Autodesk Inventor part; units mm, degrees
ref_plane "YZ Plane" through (0, 0, 0) normal (1, 0, 0) x (0, 1, 0)
ref_plane "XZ Plane" through (0, 0, 0) normal (0, 1, 0) x (-1, 0, 0)
ref_plane "XY Plane" through (0, 0, 0) normal (0, 0, 1) x (1, 0, 0)
sketch "Sketch1" plane through (0, 0, 0) normal (0, 1, 0) x (-1, 0, 0)
  line L0 (-27.94, -43.053) -> (27.94, -43.053)
  line L1 (27.94, -43.053) -> (27.94, 43.053)
  line L2 (27.94, 43.053) -> (-27.94, 43.053)
  line L3 (-27.94, 43.053) -> (-27.94, -43.053)
  line L4 (-27.94, -43.053) -> (27.94, 43.053) construction
  line L5 (27.94, -43.053) -> (-27.94, 43.053) construction
  point P0 (0, 0)
  dimension "d0" = 86.106
  dimension "d1" = 55.88
extrude "Extrusion1" add sketch "Sketch1" along normal blind 0.8
fillet "Fillet1" radius 3.9688 4 edges at (27.94, 0.4, 43.053) (27.94, 0.4, -43.053) (-27.94, 0.4, -43.053) (-27.94, 0.4, 43.053)
sketch "Sketch2" plane through (0, 0.8, 0) normal (0, 1, 0) x (1, 0, 0)
  line L0 (7.5, -73.053) -> (-7.5, -73.053)
  line L1 (-7.5, -73.053) -> (-7.5, -13.053)
  line L2 (-7.5, -13.053) -> (7.5, -13.053)
  line L3 (7.5, -13.053) -> (7.5, -73.053)
  line L4 (-23.9712, -43.053) -> (23.9713, -43.053)
  line L5 (7.5, -73.053) -> (-7.5, -13.053) construction
  line L6 (-7.5, -73.053) -> (7.5, -13.053) construction
  point P0 (0, 0)
  point P1 (0, -43.053)
  point P2 (-7.5, -43.053)
  point P3 (7.5, -43.053)
  dimension "d5" = 15
  dimension "d6" = 60
extrude "Extrusion2" cut sketch "Sketch2" against normal blind 25.4 contours L4 L1 L2 L3
fillet "Fillet2" radius 1.5875 4 edges at (-7.5, 0.4, 13.053) (7.5, 0.4, 13.053) (-7.5, 0.4, 43.053) (7.5, 0.4, 43.053)
properties part number "led_ring_cover"
Input: part model. Units: mm. Frame: model coordinates. A direction names the side the tool comes from. Give positions to 0.01 mm unless a question says otherwise; leave off trailing zeros. Write each loop counter-clockwise with the first axis right and the second up, starting at its lowest first coordinate (ties: lowest second). Pieces come first, ordered by that corner, then holes. Notation, with made-up numbers: (14, 52.5) -> (58, 52.5) arc R16 ccw to (58, 77.5) -> close; hole circle Ø1 at (64, 3.5). An arc over 180 degrees is marked (long way). Use one line per item in the form item = value. Start each with the question number.
1) Set-up query: faces 5 (the flat face through (0, 0, 1)), 6 (the cylindrical face through (-7.047, 0.394, 13.53)). Return all of +Z, -Z, +X, -X, +Y, -Y with unobstructed straight access to the full face (end or side cutting, diameter ignored); none if empty.
2) Draft query along X for faces 1 (the cylindrical face through (-7.953, 0.394, 42.576)), 2 (the cylindrical face through (-26.81, 0.41, 41.86)), 3 (the cylindrical face through (26.75, 0.41, 41.92)), 4 (the flat face through (0, 0.8, 1)). Return one class per face: pulls with the +X half, pulls with the -X half, needs draft (parallel to the pull), parting line crosses it, or undercut.
3) Ray query, probe 1 along X at (y, z) = (0.15, 35.5); probe 2 along Z at (x, y) = (-3, 0.4); probe 3 along Z at (x, y) = (-25.5, 0.5). Return the intervals inside material, ascending. Write a range as from..to.
4) Section query A-A on z = 37. Return the cut outline in (x, y), then the cut area to 3 significant figures.
5) Pin query (flat end, axial travel): pin 1 (3 mm diameter, centred on x = 7, z = 32, fed in from -Y). Return the tip coordinate at first contact, or that it passes through.
6) Section query B-B on y = 0.55. Return the cut outline in (x, z) (1 decimal).
7) Section query C-C on x = 4. Return the cut outline in (y, z), then the cut area to 3 significant figures.
Outcome:
q1.face_5 = +Z, -Z, +X, -X, -Y
q1.face_6 = +Z, +Y, -Y
q2.face_1 = undercut
q2.face_2 = pulls with the -X half
q2.face_3 = pulls with the +X half
q2.face_4 = needs draft
q3.probe_1 = -27.94..-7.5, 7.5..27.94
q3.probe_2 = -43.05..13.05
q3.probe_3 = -42.75..42.75
q4.outline = (-27.94, 0) -> (-7.5, 0) -> (-7.5, 0.8) -> (-27.94, 0.8) -> close; (7.5, 0) -> (27.94, 0) -> (27.94, 0.8) -> (7.5, 0.8) -> close
q4.area = 32.7 mm^2
q5.pin_1 = 0
q6.outline = (-27.9, -39.1) arc R4 ccw to (-24, -43.1) -> (24, -43.1) arc R4 ccw to (27.9, -39.1) -> (27.9, 39.1) arc R4 ccw to (24, 43.1) -> (9.1, 43.1) arc R1.6 ccw to (7.5, 41.5) -> (7.5, 14.6) arc R1.6 cw to (5.9, 13.1) -> (-5.9, 13.1) arc R1.6 cw to (-7.5, 14.6) -> (-7.5, 41.5) arc R1.6 ccw to (-9.1, 43.1) -> (-24, 43.1) arc R4 ccw to (-27.9, 39.1) -> close
q7.outline = (0, -43.05) -> (0.8, -43.05) -> (0.8, 13.05) -> (0, 13.05) -> close
q7.area = 44.9 mm^2
